Autodesk Inventor part; units mm, degrees
ref_plane "Work Plane1" through (-20.8033, -6.3, -5.9) normal (0, 0, 1) x (1, 0, 0)
ref_plane "YZ Plane" through (0, 0, 0) normal (1, 0, 0) x (0, 1, 0)
ref_plane "XZ Plane" through (0, 0, 0) normal (0, 1, 0) x (-1, 0, 0)
sketch "Sketch1" plane through (0, 0, 0) normal (0, 0, 1) x (1, 0, 0)
  line L0 (0.8467, -0.7217) -> (0.8467, 0.7217) construction
  line L1 (0.8467, 0.7217) -> (2.0967, 1.4434) construction
  line L2 (2.0967, 1.4434) -> (3.3467, 0.7217) construction
  line L3 (3.3467, 0.7217) -> (3.3467, -0.7217) construction
  line L4 (3.3467, -0.7217) -> (2.0967, -1.4434) construction
  line L5 (2.0967, -1.4434) -> (0.8467, -0.7217) construction
  circle A0 centre (2.0967, 0) radius 2.45 construction
  line L6 (4.8467, -1.5877) -> (3.4717, -2.3816) construction
  line L7 (15.0967, 3) -> (15.0967, -3) construction
  line L8 (-10.9033, 3) -> (-10.9033, -3) construction
  line L9 (-0.6533, 0) -> (-0.6533, 1.5877) construction
  circle A1 centre (2.0967, 0) radius 5
  circle A2 centre (2.0967, 0) radius 1.7
  line L10 (-10.9033, -3) -> (15.0967, -3)
  line L11 (-10.9033, 3) -> (15.0967, 3)
  circle A3 centre (2.0967, 0) radius 2.7
  circle A4 centre (2.0967, 0) radius 6
  circle A5 centre (2.0967, 0) radius 2.75
  point P0 (0.4719, -0.5)
  point P1 (3.7215, -0.5)
  dimension "d10" = 5.4
  dimension "d13" = 12
ref_plane "Work Plane1" through (-20.8033, -6.3, -5.9) normal (0, 0, 1) x (1, 0, 0)
extrude "Extrusion1" add sketch "Sketch1" against normal blind 4 contours A1 L10 L11 | A1 L11 A4 L10 | L11 A1 | A1 L11 A4 | L10 A4 A1 | A1 L10 | A1 L10 A4 L11 | A5
sketch "Sketch2" plane through (2.0967, 0, 0) normal (0, 0, 1) x (1, 0, 0)
  line L0 (-2, 1.5) -> (2, 1.5) construction
  arc A0 (2.5, 0) -> (2, 1.5) centre (0, 0) ccw construction
  arc A1 (-2, 1.5) -> (-2.5, 0) centre (0, 0) ccw construction
  line L1 (2, -1.5) -> (-2, -1.5) construction
  arc A2 (-2.5, 0) -> (2.5, 0) centre (0, 0) ccw construction
  line L2 (2.0248, 1.55) -> (-2.0248, 1.55) construction
  arc A3 (-2.0248, 1.55) -> (-2.55, 0) centre (0, 0) ccw construction
  arc A4 (-2.55, 0) -> (2.55, 0) centre (0, 0) ccw construction
  arc A5 (2.55, 0) -> (2.0248, 1.55) centre (0, 0) ccw construction
  line L3 (-2.0248, 1.55) -> (2.0248, 1.55) construction
  line L4 (-2.0248, 1.55) -> (2.0248, 1.55)
  line L5 (-2.0248, -1.55) -> (2.0248, -1.55)
  arc A6 (-2.0248, 1.55) -> (-2.0248, -1.55) centre (0, 0) ccw
  arc A7 (2.0248, -1.55) -> (2.0248, 1.55) centre (0, 0) ccw
  circle A8 centre (0, 0) radius 6
  point P0 (-2.0967, 0)
  dimension "d11" = 3.1
  dimension "d12" = 2.55
extrude "Extrusion2" add sketch "Sketch2" along normal blind 5
chamfer "Chamfer1" distance 1.2 angle 45 4 edges at (2.0967, 1.55, 5) (-0.4533, 0, 5) (2.0967, -1.55, 5) (4.6467, 0, 5)
sketch "Sketch3" plane through (0, 0, 0) normal (0, 1, 0) x (-1, 0, 0)
  line L0 (-4.6467, 0) -> (-4.6467, 3.8)
  line L1 (0.4533, 0) -> (0.4533, 3.8)
  line L2 (-8.0967, -4) -> (3.9033, -4)
  circle A0 centre (-2.0967, -1.5) radius 1.25
  line L3 (-8.0967, -4) -> (3.9033, -4)
  point P0 (0, 0)
  point P1 (-8.5967, 0)
  point P2 (4.4033, 0)
  dimension "d14" = 2.5
  dimension "d15" = 2.5
extrude "Extrusion3" cut sketch "Sketch3" against normal blind 10
pattern_circular "Circular Pattern1" count 3 over 360 about axis through (2.0967, 0, 0) along (0, 0, -1) of "Extrusion3"
sketch "Sketch4" plane through (0.0718, -1.55, 0) normal (0, 1, 0) x (1, 0, 0)
  line L0 (0, -3.8) -> (4.0497, -3.8)
  line L1 (-3.9752, -5) -> (8.0248, -5)
  line L2 (8.0248, 4) -> (-3.9752, 4)
  line L3 (4.0497, -3.8) -> (0, -3.8)
  line L4 (4.0497, 0) -> (4.0497, -3.8)
  line L5 (0, 0) -> (4.0497, 0)
  line L6 (0, 0) -> (0, -3.8)
  circle A0 centre (2.0248, -2.0248) radius 2.0248
  point P0 (-0.0718, 0)
  point P1 (7.732, 1.5)
  point P2 (-2.4323, 1.5)
  point P3 (0.7748, 1.5)
hole "Hole1" at (2.0967, -1.55, 2.0248) direction (0, -1, 0) diameter 2.5 end through all both
properties part number "30_Coupling_Screw_28BYJ_M3"
The listing builds one solid part. Answer for the finished solid, in the listing's coordinates (mm). A direction names the side the tool comes from. Give positions to 0.01 mm unless a question says otherwise; leave off trailing zeros. Order: outer loops, then holes, each group sorted by start corner. A loop starts at its lowest first (then second) coordinate and runs counter-clockwise, first axis right, second up. Notation, with made-up numbers: (84.5, 85) - (113.5, 85) arc R32 ccw to (113.5, 118) - close; hole circle Ø5 at (-1.75, 41). An arc over 180 degrees is marked (long way). Use one line per item in the form item = value.
1) For faces 1 (the conical face through (-0.928, 0.035, 4.275)), 2 (the flat face through (2, 2, 0)), 3 (the cylindrical face through (-0.453, -0.023, 1.873)), 4 (the cylindrical face through (3.345, -4.171, -1.445)), 5 (the cylindrical face through (5, 3, -1)), determine the directions among +Z, -Z, +X, -X, +Y, -Y from which every point of the face is accessible in a straight line to the end or side of a thin tool.
Verdict:
face_1 = +Z
face_2 = -Z
face_3 = +Z, -Z
face_4 = -Y
face_5 = none
2) Find section B-B on z = -1.5. Determine the outline of the cut face in (x, y).
Verdict:
outline = (-3.61, 1.85) arc R6 ccw to (0.85, -5.87) - (0.85, -2.39) arc R2.7 cw to (-0.6, 0.11) - close; (-2.36, 4.02) - (0.65, 2.28) arc R2.7 cw to (3.54, 2.28) - (6.55, 4.02) arc R6 ccw to start; (3.35, -5.87) arc R6 ccw to (7.8, 1.85) - (4.79, 0.11) arc R2.7 cw to (3.35, -2.39) - close
3) Each of these flat-tipped pins is pushed along its axis until it touches: pin 1 (4 mm diameter, centred on y = 3, z = 2.5, fed in from +X); pin 2 (5 mm diameter, centred on x = 2.1, y = 0, fed in from -Z); pin 3 (2 mm diameter, centred on x = 2.1, z = 2.02, fed in from +Y). Where does it stop, or does it pass through?
Verdict:
pin_1 = 8.01
pin_2 = 0
pin_3 = through
4) The mould has two halves that part along X. Classify faces 6 (the cylindrical face through (4.87, 5.32, 0.44)), 7 (the flat face through (2, 3, 5)), 8 (the flat face through (2.06, -2.14, 4.39)), 9 (the conical face through (5.122, -0.035, 4.275)): released by +X, released by -X, zero draft, split by the parting line, or undercut.
Verdict:
face_6 = split by the parting line
face_7 = zero draft
face_8 = undercut
face_9 = undercut
5) Find section A-A on z = 1.75. Determine the outline of the cut face in (x, y), and give its area (3 significant figures).
Verdict:
outline = (0.07, -1.55) arc R2.55 cw to (0.07, 1.55) - (0.88, 1.55) - (0.88, 5.87) arc R6 ccw to (0.88, -5.87) - (0.88, -1.55) - close; (3.32, -5.87) arc R6 ccw to (3.32, 5.87) - (3.32, 1.55) - (4.12, 1.55) arc R2.55 cw to (4.12, -1.55) - (3.32, -1.55) - close
area = 76.8 mm^2
6) Consider probe 1 along Z at (x, y) = (3, -4.75); probe 2 along Y at (x, z) = (0.75, 3.5); probe 3 along X at (y, z) = (1.5, -1). Determine where each line is inside the solid, lowest interval first. Write a range as [from, to].
Verdict:
probe_1 = [-4, -2.36], [-0.64, 1.16], [2.89, 5]
probe_2 = [-5.85, -1.55], [1.55, 5.85]
probe_3 = [-3.71, -2.79], [6.99, 7.91]
7) Find section D-D on y = -5. Determine the outline of the cut face in (x, z).
Verdict:
outline = (-1.22, -4) - (5.41, -4) - (5.41, 5) - (-1.22, 5) - close; hole circle Ø2.5 at (2.1, -1.5); hole circle Ø2.5 at (2.1, 2.02)
8) Find section C-C on y = -3.25. Determine the outline of the cut face in (x, z).
Verdict:
outline = (-2.95, -4) - (7.14, -4) - (7.14, 5) - (-2.95, 5) - close; hole circle Ø2.5 at (2.1, -1.5); hole circle Ø2.5 at (2.1, 2.02)
